from build123d import *

# Parameters (mm, degrees)
F3_W        = 1.8414998049
F3_H        = 12.7
F3_W_2      = 12.7
F3_H_2      = 1.8414998049
F1_FACE_R   = 6.985
F1_FACE_R_2 = 2.54
F4_DEPTH    = 59.8805
F5_DEPTH    = 12.7


with BuildPart() as f1:
    # F0 (on Front) → F1 (revolve)
    with BuildSketch(Plane.XZ):
        with BuildLine():
            Line((-139.7, 0), (0, 0))
            Line((0, 0), (0, 1.905))
            ThreePointArc((0, 1.905), (-1.8598719395, 6.3951280605), (-6.35, 8.255))
            Line((-6.35, 8.255), (-39.2910341604, 8.255))
            ThreePointArc((-39.2910341604, 8.255), (-39.9260341604, 8.0848522628), (-40.3908864232, 7.62))
            ThreePointArc((-40.3908864232, 7.62), (-46.99, 3.81), (-53.5891135768, 7.62))
            ThreePointArc((-53.5891135768, 7.62), (-54.0539658396, 8.0848522628), (-54.6889658396, 8.255))
            Line((-54.6889658396, 8.255), (-55.88, 8.255))
            ThreePointArc((-55.88, 8.255), (-56.7780256121, 7.8830256121), (-57.15, 6.985))
            Line((-57.15, 6.985), (-57.15, 2.54))
            Line((-57.15, 2.54), (-139.7, 2.54))
            Line((-139.7, 2.54), (-139.7, 0))
        make_face()
    revolve(axis=Axis((31.713694334, 0, 0), (-1, 0, 0)))

    # F3 (on Right) + F1_face (on face) → F4 (cut)
    with BuildSketch(Plane.YZ):
        with Locations((7.9057499024, 0)):
            Rectangle(F3_W, F3_H)
        with Locations((0, 7.9057499024)):
            Rectangle(F3_W_2, F3_H_2)
        with Locations((-7.9057499024, 0)):
            Rectangle(F3_W, F3_H)
        with Locations((0, -7.9057499024)):
            Rectangle(F3_W_2, F3_H_2)
    with BuildSketch(Plane(origin=(-57.15, 0, 0), x_dir=(0, -1, 0), z_dir=(-1, 0, 0))):
        Circle(F1_FACE_R)
        Circle(F1_FACE_R_2, mode=Mode.SUBTRACT)
    extrude(amount=-F4_DEPTH, dir=(1, 0, 0), mode=Mode.SUBTRACT)

    # F2 (on Front) → F5 (cut, symmetric)
    with BuildSketch(Plane.XZ):
        Polygon((-139.7, 2.54), (-139.7, 0.3175), (-118.5543250005, 2.54), align=None)
        Polygon((-139.7, -0.3175), (-139.7, -2.54), (-118.5543250005, -2.54), align=None)
    extrude(amount=F5_DEPTH, both=True, mode=Mode.SUBTRACT)


solid = f1.part
Geometry check sheet. Reference: the model listing, model coordinates, mm. A direction names the side the tool comes from. Round coordinates to 2 decimals unless told otherwise and drop trailing zeros. Loops run counter-clockwise (first coordinate to the right, second up) from the corner with the lowest first, then second, coordinate; pieces in that order, holes last. Notation, with made-up numbers: (18.5, 44) - (47.5, 44) arc R15 cw to (47.5, 48) - close; hole circle Ø4 at (71, 73). An arc over 180 degrees is marked (long way). One line per question, with ' | ' between items. Start each with the question number.
1. Cross-section at B-B on x = -46. Record the cut outline in (y, z).
2. Tool access check on faces 1 (the face through (-89.831, 0.763, 2.423)), 2 (the face through (-23.051, 5.819, 5.855)). Record the directions out of +Z, -Z, +X, -X, +Y, -Y that give a thin tool (end or side, any length) a straight path to the whole face; none if there is none.
3. Scan lines: line 1 (Z direction, x = -89.5, y = 0); line 2 (X direction, y = 5.5, z = 4); line 3 (X direction, y = 3.75, z = 5). Record each from-to range of solid material in increasing order. Write a range as [from, to].
4. Depth check by flat-ended pin: pin 1 (2 mm diameter, centred on x = -111.5, z = -1, fed in from -Y); pin 2 (1 mm diameter, centred on x = -90.5, z = -1.5, fed in from +Y); pin 3 (3 mm diameter, centred on x = -74, y = -4.5, fed in from +Z); pin 4 (6 mm diameter, centred on x = -49.5, y = 2.5, fed in from +Z). Enter the tip coordinate at first touch or a pass-through.
5. Cross-section at A-A on x = -88. Record the cut outline in (y, z), then the cut area to 3 significant figures.
Taken from the geometry:
1) outline: circle Ø7.75 at (0, 0)
2) face 1: -X | face 2: +Z, +X, -X, +Y
3) line 1: [-2.54, 2.54] | line 2: [-57.15, -53.04], [-40.94, -2.31] | line 3: [-57.15, -52.58], [-41.4, -1.72]
4) pin 1: y = -2.54 | pin 2: y = 2.33 | pin 3: through | pin 4: z = 5.81
5) outline: circle Ø5.08 at (0, 0) | area: 20.3 mm²
